The model under review builds one solid part; all positions refer to its coordinate system, in mm. Coordinates: 2 decimals unless noted, no trailing zeros. Order: outer loops, then holes, each group sorted by start corner. A loop starts at its lowest first (then second) coordinate and runs counter-clockwise, first axis right, second up. Notation, with made-up numbers: M -27.75,15.25 L -16.75,15.25 A35 ccw -16.75,51.25 Z; hole C 10.5,2 d4. An arc over 180 degrees is marked long. One line per item, written item: value.
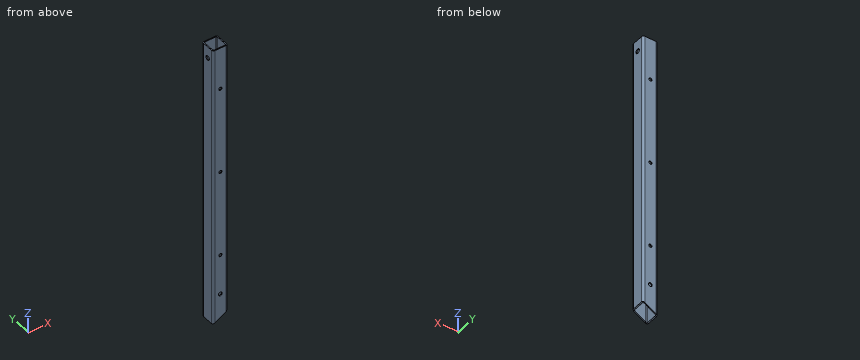
Autodesk Inventor part; units mm, degrees
ref_plane "YZ Plane" through (0, 0, 0) normal (1, 0, 0) x (0, 1, 0)
ref_plane "XZ Plane" through (0, 0, 0) normal (0, 1, 0) x (-1, 0, 0)
ref_plane "XY Plane" through (0, 0, 0) normal (0, 0, 1) x (1, 0, 0)
sketch "Sketch1" plane through (0, 0, 0) normal (0, 0, 1) x (1, 0, 0)
  line L0 (3.7363, 0) -> (22.7863, 0)
  line L1 (25.9613, 3.175) -> (25.9613, 22.225)
  line L2 (22.7863, 25.4) -> (3.7363, 25.4)
  line L3 (0.5613, 22.225) -> (0.5613, 3.175)
  arc A0 (3.7363, 25.4) -> (0.5613, 22.225) centre (3.7363, 22.225) ccw
  arc A1 (0.5613, 3.175) -> (3.7363, 0) centre (3.7363, 3.175) ccw
  arc A2 (22.7863, 0) -> (25.9613, 3.175) centre (22.7863, 3.175) ccw
  arc A3 (25.9613, 22.225) -> (22.7863, 25.4) centre (22.7863, 22.225) ccw
  line L4 (3.7363, 23.749) -> (22.7863, 23.749)
  arc A4 (24.3103, 22.225) -> (22.7863, 23.749) centre (22.7863, 22.225) ccw
  line L5 (24.3103, 22.225) -> (24.3103, 3.175)
  arc A5 (22.7863, 1.651) -> (24.3103, 3.175) centre (22.7863, 3.175) ccw
  line L6 (22.7863, 1.651) -> (3.7363, 1.651)
  arc A6 (2.2123, 3.175) -> (3.7363, 1.651) centre (3.7363, 3.175) ccw
  line L7 (2.2123, 3.175) -> (2.2123, 22.225)
  arc A7 (3.7363, 23.749) -> (2.2123, 22.225) centre (3.7363, 22.225) ccw
  point P0 (0, 0)
  point P1 (0.5613, 0)
  point P2 (25.9613, 0)
  point P3 (0.5613, 25.4)
  dimension "d0" = 25.4
  dimension "d2" = 25.4
  dimension "d3" = 3.175
  dimension "d4" = 1.651
extrude "tube" add sketch "Sketch1" along normal blind 520.3
sketch "Sketch11" plane through (3.7363, 25.4, 0) normal (0, 1, 0) x (1, 0, 0)
  line L0 (19.05, 0) -> (0, 0)
  circle A0 centre (9.525, -20) radius 2.8743
  point P0 (-3.7363, 0)
  dimension "d83" = 20
hole "centerHole_cutOff" at (13.2613, 25.4, 20) direction (0, -1, 0) diameter 6.35 end through all
sketch "Sketch12" plane through (3.7363, 25.4, 0) normal (0, 1, 0) x (1, 0, 0)
  circle A0 centre (9.525, -20) radius 3.175
  circle A1 centre (9.525, -77) radius 2.5235
  point P0 (-3.7363, 0)
  dimension "d91" = 57
hole "collarHole" at (13.2613, 25.4, 77) direction (0, -1, 0) diameter 6.6 end through all
sketch "Sketch8" plane through (3.7363, 25.4, 520.3) normal (0, 1, 0) x (1, 0, 0)
  line L0 (0, 520.3) -> (0, 0)
  circle A0 centre (9.525, 73.3) radius 1.5875
  circle A1 centre (9.525, 223.3) radius 1.5875
  circle A2 centre (9.525, 373.3) radius 1.5875
  circle A3 centre (9.525, 500.3) radius 3.175
  point P0 (0, 518.1689)
  point P1 (-3.7363, 520.3)
  dimension "d43" = 3.175
  dimension "d47" = 150
  dimension "d99" = 127
hole "armAttach" at (13.2613, 25.4, 447) at (13.2613, 25.4, 297) at (13.2613, 25.4, 147) direction (0, -1, 0) diameter 5.5 end through all
sketch "Sketch6" plane through (25.9613, 3.175, 520.3) normal (1, 0, 0) x (0, 0, -1)
  line L0 (0, 0) -> (0, 19.05)
  circle A0 centre (20, 9.525) radius 2.9685
  point P0 (520.3, -3.175)
  dimension "d27" = 20
hole "ropeAttach" at (25.9613, 12.7, 500.3) direction (-1, 0, 0) diameter 8 end through all
sketch "Sketch13" plane through (3.7363, 25.4, 0) normal (0, 1, 0) x (1, 0, 0)
  circle A0 centre (9.525, -20) radius 3.175
  line L0 (9.525, -20) -> (9.525, -34.6812) construction
  line L1 (-12.9518, -21.6531) -> (31.0422, -47.0531)
  line L2 (0, -34.6812) -> (50.8, -34.6812) construction
  line L3 (-12.9518, 4.6365) -> (31.0422, 4.6365)
  line L4 (31.0422, -47.0531) -> (31.0422, 4.6365)
  line L5 (-12.9518, 4.6365) -> (-12.9518, -21.6531)
  point P0 (-3.7363, 0)
  dimension "d100" = 14.6812
  dimension "d101" = 50.8
  dimension "d102" = 30
extrude "angledEnd" cut sketch "Sketch13" against normal blind 50.8
equation "\"tube\" = 25.4"
properties part number "2f2ax1" material "Steel"
(1) We need section B-B, the plane z = 500.3. State the section outline as (x, y) points (3 decimals).
Geometry results:
outline: M 0.561,3.175 A3.175 ccw 3.736,0 L 22.786,0 A3.175 ccw 25.961,3.175 L 25.961,8.7 L 24.31,8.7 L 24.31,3.175 A1.524 cw 22.786,1.651 L 3.736,1.651 A1.524 cw 2.212,3.175 L 2.212,8.7 L 0.561,8.7 Z; M 0.561,16.7 L 2.212,16.7 L 2.212,22.225 A1.524 cw 3.736,23.749 L 22.786,23.749 A1.524 cw 24.31,22.225 L 24.31,16.7 L 25.961,16.7 L 25.961,22.225 A3.175 ccw 22.786,25.4 L 3.736,25.4 A3.175 ccw 0.561,22.225 Z
(2) For L1, parallel to Y at x = 14.25, z = 176; L2, parallel to X at y = 20.5, z = 314; L3, parallel to Z at x = 15.25, y = 24.25, list the stretches that pass through material, from the lowest coordinate up.
Geometry results:
L1: y = 0 to 1.65, 23.75 to 25.4
L2: x = 0.56 to 2.21, 24.31 to 25.96
L3: z = 35.78 to 74.37, 79.63 to 145.1, 148.9 to 295.1, 298.9 to 445.1, 448.9 to 520.3
(3) We need section A-A, the plane z = 158.5. State the section outline as (x, y) points (3 decimals), plus the area to 3 significant figures.
Geometry results:
outline: M 0.561,3.175 A3.175 ccw 3.736,0 L 22.786,0 A3.175 ccw 25.961,3.175 L 25.961,22.225 A3.175 ccw 22.786,25.4 L 3.736,25.4 A3.175 ccw 0.561,22.225 Z; hole M 2.212,3.175 A1.524 ccw 3.736,1.651 L 22.786,1.651 A1.524 ccw 24.31,3.175 L 24.31,22.225 A1.524 ccw 22.786,23.749 L 3.736,23.749 A1.524 ccw 2.212,22.225 Z
area: 150 mm2
